Could you check a few things on this model? Use its own coordinates, in mm. A direction names the side the tool comes from. Round coordinates to 2 decimals unless told otherwise and drop trailing zeros. Loops run counter-clockwise (first coordinate to the right, second up) from the corner with the lowest first, then second, coordinate; pieces in that order, holes last. Notation, with made-up numbers: M -5,5 L 53,5 A20 ccw 53,24 Z; hole C 45,-0.5 d10. An arc over 180 degrees is marked long. One line per item, written item: value. Start each with the question number.
Q1. Which directions (+Z, -Z, +X, -X, +Y, -Y) give clear straight access to the entire face, cutting with the end or side of a thin tool? Please do faces 1 (the face through (0, 6.731, 108)), 2 (the face through (5, -8, 108)), 3 (the face through (0, 8.66, 108)), 4 (the face through (-5, -8, 108)).
Q2. Please list where these lines run through material, in increasing order: line 1 along X through (y, z) = (7.8, 115); line 2 along Z through (x, y) = (-2, -1.75); line 3 along X through (y, z) = (-0.25, 53).
Q3. Thinking about a two-plate mould opening in Y: for faces 5 (the face through (4, -8, 118)), 6 (the face through (0, -8.66, 108)), 7 (the face through (0, 0, 100)), 8 (the face through (0, -6.731, 108)), which applies, released by +Y, released by -Y, zero draft, split by the parting line, or undercut?
Q4. Imagine slicing it at C-C (x = 8.75). Please give me the cut outline in (y, z), then the cut area to 3 significant figures.
Q5. Imagine slicing it at A-A (y = 0). Please give me the cut outline in (x, z), then the cut area to 3 significant figures.
Q6. Imagine slicing it at B-B (z = 93.5). Please give me the cut outline in (x, y), then the cut area to 3 significant figures.
Q7. I'm going to push flat-ended pins straight in: pin 1 Ø8 at (x, z) = (0.5, 109.5) entering from -Y; pin 2 Ø4 at (y, z) = (-6, 29) entering from +X; pin 3 Ø2.5 at (y, z) = (7.5, 104) entering from +X; pin 4 Ø5.5 at (x, z) = (0, 115) entering from +Y. Where does each tip first touch, or does it pass through?
from build123d import *

# Parameters (mm, degrees)
SKETCH1_R           = 10
BOSS_EXTRUDE1_DEPTH = 100
SKETCH3_W           = 10
SKETCH3_H           = 1.929631273
BOSS_EXTRUDE3_DEPTH = 20
SKETCH4_R           = 3
CUT_EXTRUDE1_DEPTH  = 122.853211204
FILLET2_R           = 5
FILLET3_R           = 1.35
SKETCH7_R           = 1.5
BOSS_EXTRUDE4_DEPTH = 13


# Some blends are built 0.0001 mm under size
with BuildPart() as part:
    # Sketch1 → Boss-Extrude1 (new body)
    with BuildSketch(Plane(origin=(0, 0, 0), x_dir=(0, 1, 0), z_dir=(0, 0, 1))):
        with Locations(Location((0, 0, 0), (0, 0, 270))):
            Circle(SKETCH1_R)
    extrude(amount=BOSS_EXTRUDE1_DEPTH)

    # Sketch3 → Boss-Extrude3 (add)
    with BuildSketch(Plane.XY.offset(100)):
        with Locations((0, 7.695438402)):
            Rectangle(SKETCH3_W, SKETCH3_H)
        with Locations((0, -7.695438402)):
            Rectangle(SKETCH3_W, SKETCH3_H)
    extrude(amount=BOSS_EXTRUDE3_DEPTH)

    # Sketch4 → Cut-Extrude1 (cut, through all)
    with BuildSketch(Plane.XZ.offset(8.660254038)):
        with Locations(Location((0, 115, 0), (0, 0, 270))):
            Circle(SKETCH4_R)
    extrude(amount=-CUT_EXTRUDE1_DEPTH, mode=Mode.SUBTRACT)

    # Fillet2
    fillet2_edges = [part.edges().sort_by_distance(p)[0] for p in [
        (-5, 7.695438402, 120),
        (5, 7.695438402, 120),
        (-5, -7.695438402, 120),
        (5, -7.695438402, 120),
    ]]
    fillet(fillet2_edges, radius=FILLET2_R - 0.0001)  # a hair under: the kernel refuses the full size

    # Fillet3
    # the kernel refuses this fillet: 1.35 mm, written as the material it adds along each edge
    with BuildSketch(Plane(origin=(-5, -6.730622765, 100), x_dir=(0, 0, 1), z_dir=(1, 0, 0)), Plane(origin=(-5, 6.730622765, 100), x_dir=(0, -1, 0), z_dir=(1, 0, 0))) as fillet3_piece_1:
        with BuildLine():
            CenterArc((FILLET3_R, -FILLET3_R), FILLET3_R, 90, 90)
            Line((0, -FILLET3_R), (0, 0))
            Line((0, 0), (FILLET3_R, 0))
        make_face()
    extrude(amount=10)
    with BuildSketch(Plane(origin=(5, 8.660254038, 100), x_dir=(0, 1, 0), z_dir=(-1, 0, 0))) as fillet3_piece_2_section:
        with BuildLine():
            CenterArc((FILLET3_R, -FILLET3_R), FILLET3_R, 90, 90)
            Line((0, -FILLET3_R), (0, 0))
            Line((0, 0), (FILLET3_R, 0))
        make_face()
    fillet3_piece_2 = extrude(amount=10, mode=Mode.PRIVATE)
    fillet3_piece_2 = fillet3_piece_2 & Plane(origin=(0, 0, 100.331461228), x_dir=(1, 0, 0), z_dir=(0, 0, -1)) * Cylinder(10, 26, mode=Mode.PRIVATE)
    add(fillet3_piece_2)
    with BuildSketch(Plane(origin=(5, -8.660254038, 100), x_dir=(0, 0, 1), z_dir=(-1, 0, 0))) as fillet3_piece_3_section:
        with BuildLine():
            CenterArc((FILLET3_R, -FILLET3_R), FILLET3_R, 90, 90)
            Line((0, -FILLET3_R), (0, 0))
            Line((0, 0), (FILLET3_R, 0))
        make_face()
    fillet3_piece_3 = extrude(amount=10, mode=Mode.PRIVATE)
    fillet3_piece_3 = fillet3_piece_3 & Plane(origin=(0, 0, 100.331460994), x_dir=(1, 0, 0), z_dir=(0, 0, -1)) * Cylinder(10, 26, mode=Mode.PRIVATE)
    add(fillet3_piece_3)

    # Sketch7 → Boss-Extrude4 (add)
    with BuildSketch(Plane(origin=(0, 0, 0), x_dir=(-1, 0, 0), z_dir=(0, 1, 0))):
        with Locations(Location((0, 11.098495107, 0), (0, 0, 270))):
            Circle(SKETCH7_R)
    extrude(amount=BOSS_EXTRUDE4_DEPTH)


solid = part.part
Report:
1. face 1: +Z, +X, -X
1. face 2: +Z, +X, +Y, -Y
1. face 3: +Z, +X, -X, +Y
1. face 4: +Z, -X, +Y, -Y
2. line 1: x = -5 to -3, 3 to 5
2. line 2: z = 0 to 100
2. line 3: x = -10 to 10
3. face 5: zero draft
3. face 6: released by -Y
3. face 7: undercut
3. face 8: undercut
4. outline: M -4.84,0 L 4.84,0 L 4.84,100 L -4.84,100 Z
4. area: 968 mm²
5. outline: M -10,0 L 10,0 L 10,100 L -10,100 Z
5. area: 2,000 mm²
6. outline: C 0,0 d20
6. area: 314 mm²
7. pin 1: stops at y = -8.66
7. pin 2: stops at x = 9.17
7. pin 3: stops at x = 5
7. pin 4: passes through
